Read the model definition and answer for the solid it produces. Units are mm, in the model's axes. A direction names the side the tool comes from. Give positions to 0.01 mm unless a question says otherwise; leave off trailing zeros. Order: outer loops, then holes, each group sorted by start corner. A loop starts at its lowest first (then second) coordinate and runs counter-clockwise, first axis right, second up. Notation, with made-up numbers: (48.5, 16) - (99.5, 16) arc R25 ccw to (99.5, 45) - close; hole circle Ø7 at (35, 11). An arc over 180 degrees is marked (long way). Use a Markdown table: item, result. Add a question column.
1. A cutting plane is placed at B-B on z = 20. Determine the outline of the cut face in (x, y).
2. A cutting plane is placed at D-D on x = 18. State how many separate pieces and enclosed holes the cut face has, and give its area (3 significant figures).
3. For a pull along Z with two mould halves and no side action, classify faces 4 (the flat face through (23.125, 25.439, 80.578)), 5 (the flat face through (43.46, 57.95, 42.32)), 6 (the flat face through (43, 0, 49)) as released by +Z, released by -Z, zero draft, split by the parting line, or undercut.
4. Consider L1, parallel to Z at x = 56.5, y = 26; L2, parallel to X at y = 34.5, z = 28; L3, parallel to X at y = 97, z = 6. Determine where each line is inside the solid, lowest interval first.
5. Which of the six approach directions +Z, -Z, +X, -X, +Y, -Y give full straight-line access (tool end or side, diameter ignored) to faces 1 (the flat face through (49, 114.3, 49)), 2 (the flat face through (52, 6.35, 52)), 3 (the flat face through (23.125, 93.511, 80.578))?
6. A cutting plane is placed at A-A on y = 35. Determine the outline of the cut face in (x, z) (3 decimals), and give its area (3 significant figures).
7. A cutting plane is placed at C-C on x = 61. Determine the outline of the cut face in (y, z).
8. Flat-ended cylindrical pins translate along their axes: P1, Ø3, axis at y = 90, z = 59.5, coming from the +X side; P2, Ø4, axis at x = 48, y = 93, coming from the +Z side; P3, Ø8, axis at x = 14.5, y = 49, coming from the +Z side. Find the tip coordinate at first contact, or state that the pin passes through.
```python
from build123d import *

# Parameters (mm, degrees)
SKETCH1_R           = 85.725
BOSS_EXTRUDE1_DEPTH = 114.3
CUT_EXTRUDE1_DEPTH  = 152.4
SKETCH4_R           = 2.778125
CUT_EXTRUDE2_DEPTH  = 12.7
SKETCH5_R           = 6.985
CUT_EXTRUDE3_DEPTH  = 6.35


with BuildPart() as part:
    # Sketch1 → Boss-Extrude1 (new body)
    with BuildSketch(Plane(origin=(0, 0, 0), x_dir=(1, 0, 0), z_dir=(0, 1, 0))):
        Circle(SKETCH1_R)
    extrude(amount=BOSS_EXTRUDE1_DEPTH)

    # Sketch2 → Cut-Extrude1 (cut)
    with BuildSketch(Plane(origin=(0, 114.3, 0), x_dir=(1, 0, 0), z_dir=(0, 1, 0))):
        Polygon((85.724933621, -0.10668), (0, -85.725), (-45.627504124, -96.719379999), (-137.428949547, 46.173941299), (19.12530113, 101.910533163), (109.833872203, 30.600481808), align=None)
    extrude(amount=-CUT_EXTRUDE1_DEPTH, mode=Mode.SUBTRACT)

    # Sketch4 → Cut-Extrude2 (cut)
    with BuildSketch(Plane(origin=(42.862466811, 0, 42.91584), x_dir=(-0.707546622, 0, 0.706666667), z_dir=(-0.706666667, 0, -0.707546622))):
        with Locations((40.618496709, 93.472)):
            Circle(SKETCH4_R)
        with Locations((-4.847503262, 93.472)):
            Circle(SKETCH4_R)
        with Locations((-4.847503262, 25.4)):
            Circle(SKETCH4_R)
        with Locations((40.618496632, 25.4)):
            Circle(SKETCH4_R)
    extrude(amount=-CUT_EXTRUDE2_DEPTH, mode=Mode.SUBTRACT)

    # Sketch5 → Cut-Extrude3 (cut)
    with BuildSketch(Plane(origin=(0, 0, 0), x_dir=(-1, 0, 0), z_dir=(0, -1, 0))):
        with Locations((-51.837133477, -51.901682099)):
            Circle(SKETCH5_R)
    extrude(amount=-CUT_EXTRUDE3_DEPTH, mode=Mode.SUBTRACT)


solid = part.part
```
Output values:
| question | item | result |
|---|---|---|
| 1 | outline | (65.81, 0) - (83.36, 0) - (83.36, 114.3) - (65.81, 114.3) - close |
| 2 | separate pieces | 1 |
| 2 | enclosed holes | 2 |
| 2 | area | 1,770 mm² |
| 3 | face 4 | undercut |
| 3 | face 5 | released by -Z |
| 3 | face 6 | zero draft |
| 4 | L1 | 29.3 to 45.87, 47.24 to 64.47 |
| 4 | L2 | 57.8 to 81.02 |
| 4 | L3 | 79.82 to 85.51 |
| 5 | face 1 | +Z, -Z, +X, -X, +Y |
| 5 | face 2 | -Y |
| 5 | face 3 | none |
| 6 | outline | (0, 85.725) - (85.725, 0.107) arc R85.725 ccw to start |
| 6 | area | 2,090 mm² |
| 7 | outline | (0, 24.8) - (114.3, 24.8) - (114.3, 60.23) - (0, 60.23) - close |
| 8 | P1 | x = 63.13 |
| 8 | P2 | z = 72.34 |
| 8 | P3 | z = 85.08 |
